Source: CAD feature listing. Evaluate the final solid. Frame: model axes, mm. Face numbers are marked on the shaded views. A direction names the side the tool comes from. Round coordinates to 2 decimals unless told otherwise and drop trailing zeros. Loops run counter-clockwise (first coordinate to the right, second up) from the corner with the lowest first, then second, coordinate; pieces in that order, holes last. Notation, with made-up numbers: M 71.5,77 L 102.5,77 A20 ccw 102.5,107 Z; hole C -4,-34 d2. An arc over 180 degrees is marked long. One line per item, written item: value.
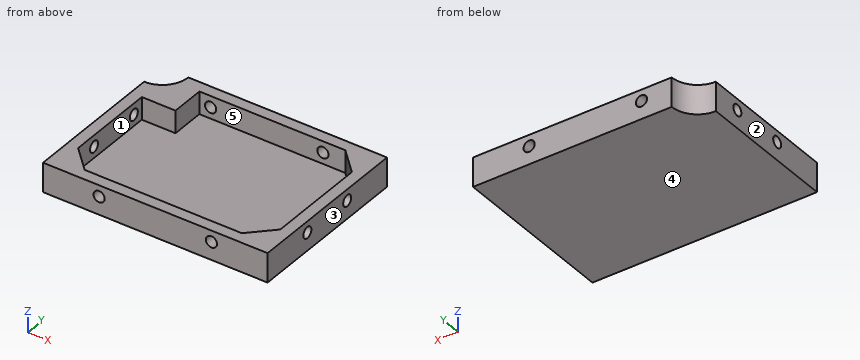
from build123d import *

# Parameters (mm, degrees)
BOSS_EXTRU_1_DEPTH        = 13
COQUE1_T                  = -5
COQUE1_THICKNESS_2_FACE_W = 90
COQUE1_THICKNESS_2_FACE_H = 65
COQUE1_THICKNESS_2_DEPTH  = 2
ENL_V_MAT_EXTRU_1_REACH   = 110.96
ESQUISSE2_R               = 2.5
ENL_V_MAT_EXTRU_2_REACH   = 95.396
ESQUISSE3_R               = 2.5
ESQUISSE4_W               = 15
ESQUISSE4_H               = 15
BOSS_EXTRU_2_DEPTH        = 10
ESQUISSE6_R               = 11.5
ENL_V_MAT_EXTRU_4_DEPTH   = 13


with BuildPart() as part:
    # Esquisse1 → Boss.-Extru.1 (new body)
    with BuildSketch(Plane.XY):
        Polygon((44.118436308, 33.728448276), (54.118436308, 33.728448276), (54.118436308, 23.728448276), (54.118436308, -41.271551724), (-45.881563692, -41.271551724), (-45.881563692, 33.728448276), align=None)
    extrude(amount=BOSS_EXTRU_1_DEPTH)

    # Coque1
    coque1_openings = [part.faces().sort_by_distance(p)[0] for p in [
        (4.118436308, -3.771551724, 13),
    ]]
    offset(amount=COQUE1_T, openings=coque1_openings, kind=Kind.INTERSECTION)

    # Coque1 thickness 2 face (on inner face of the shell) → Coque1 thickness 2 (cut)
    with BuildSketch(Plane(origin=(4.118436308, -3.771551724, 5), x_dir=(-1, 0, 0), z_dir=(0, 0, -1))):
        Rectangle(COQUE1_THICKNESS_2_FACE_W, COQUE1_THICKNESS_2_FACE_H)
    extrude(amount=COQUE1_THICKNESS_2_DEPTH, mode=Mode.SUBTRACT)

    # Enlèv. mat.-Extru.1: up to this face of the body (flat: up to its plane)
    enl_v_mat_extru_1_end = Plane(part.part.faces().sort_by_distance((54.118436308, -3.771551724, 6.5))[0])
    # Esquisse2 → Enlèv. mat.-Extru.1 (cut, up to the picked face)
    with BuildSketch(Plane.ZY.offset(45.881563692), mode=Mode.PRIVATE) as enl_v_mat_extru_1_sk1:
        with Locations(Location((8, -16.271551724, 0), (0, 0, 270))):
            Circle(ESQUISSE2_R)
    enl_v_mat_extru_1_tool1 = split(extrude(enl_v_mat_extru_1_sk1.sketch, amount=-ENL_V_MAT_EXTRU_1_REACH, mode=Mode.PRIVATE), bisect_by=enl_v_mat_extru_1_end, keep=Keep.BOTH, mode=Mode.PRIVATE)
    # Esquisse2 → Enlèv. mat.-Extru.1 (cut, up to the picked face)
    with BuildSketch(Plane.ZY.offset(45.881563692), mode=Mode.PRIVATE) as enl_v_mat_extru_1_sk2:
        with Locations(Location((8, 8.728448276, 0), (0, 0, 270))):
            Circle(ESQUISSE2_R)
    enl_v_mat_extru_1_tool2 = split(extrude(enl_v_mat_extru_1_sk2.sketch, amount=-ENL_V_MAT_EXTRU_1_REACH, mode=Mode.PRIVATE), bisect_by=enl_v_mat_extru_1_end, keep=Keep.BOTH, mode=Mode.PRIVATE)
    add(enl_v_mat_extru_1_tool1.solids().sort_by(Axis((-45.881564, -16.271552, 8), (1, 0, 0)))[0], mode=Mode.SUBTRACT)
    add(enl_v_mat_extru_1_tool2.solids().sort_by(Axis((-45.881564, 8.728448, 8), (1, 0, 0)))[0], mode=Mode.SUBTRACT)

    # Enlèv. mat.-Extru.2: up to this face of the body (flat: up to its plane)
    enl_v_mat_extru_2_end = Plane(part.part.faces().sort_by_distance((4.118436308, 33.728448276, 6.5))[0])
    # Esquisse3 → Enlèv. mat.-Extru.2 (cut, up to the picked face)
    with BuildSketch(Plane.XZ.offset(41.271551724), mode=Mode.PRIVATE) as enl_v_mat_extru_2_sk1:
        with Locations(Location((-20.881563692, 8, 0), (0, 0, 270))):
            Circle(ESQUISSE3_R)
    enl_v_mat_extru_2_tool1 = split(extrude(enl_v_mat_extru_2_sk1.sketch, amount=-ENL_V_MAT_EXTRU_2_REACH, mode=Mode.PRIVATE), bisect_by=enl_v_mat_extru_2_end, keep=Keep.BOTH, mode=Mode.PRIVATE)
    # Esquisse3 → Enlèv. mat.-Extru.2 (cut, up to the picked face)
    with BuildSketch(Plane.XZ.offset(41.271551724), mode=Mode.PRIVATE) as enl_v_mat_extru_2_sk2:
        with Locations(Location((29.118436308, 8, 0), (0, 0, 270))):
            Circle(ESQUISSE3_R)
    enl_v_mat_extru_2_tool2 = split(extrude(enl_v_mat_extru_2_sk2.sketch, amount=-ENL_V_MAT_EXTRU_2_REACH, mode=Mode.PRIVATE), bisect_by=enl_v_mat_extru_2_end, keep=Keep.BOTH, mode=Mode.PRIVATE)
    add(enl_v_mat_extru_2_tool1.solids().sort_by(Axis((-20.881564, -41.271552, 8), (0, 1, 0)))[0], mode=Mode.SUBTRACT)
    add(enl_v_mat_extru_2_tool2.solids().sort_by(Axis((29.118436, -41.271552, 8), (0, 1, 0)))[0], mode=Mode.SUBTRACT)

    # Esquisse4 → Boss.-Extru.2 (add)
    with BuildSketch(Plane.XY.offset(3)):
        Polygon((-30.881563692, -36.271551724), (-40.881563692, -26.271551724), (-40.881563692, -36.271551724), align=None)
        Polygon((49.118436308, 28.728448276), (49.118436308, 18.728448276), (39.118436308, 28.728448276), align=None)
        Polygon((49.118436308, -36.271551724), (49.118436308, -26.271551724), (39.118436308, -36.271551724), align=None)
        with Locations((-33.381563692, 21.228448276)):
            Rectangle(ESQUISSE4_W, ESQUISSE4_H)
    extrude(amount=BOSS_EXTRU_2_DEPTH)

    # Esquisse6 → Enlèv. mat.-Extru.4 (cut)
    with BuildSketch(Plane.XY.offset(13)):
        with Locations((-45.881563692, 33.728448276)):
            Circle(ESQUISSE6_R)
    extrude(amount=-ENL_V_MAT_EXTRU_4_DEPTH, mode=Mode.SUBTRACT)


solid = part.part
1. Reachability of the marked faces 4 and 5 from +Z, -Z, +X, -X, +Y, -Y: full face, straight path, thin tool, end or side. Return the list, or none.
Report:
face 4: -Z, +X, -X, +Y, -Y
face 5: +Z
2. Section query C-C (y = -7.5). Return the cut outline in (x, z), and give its area (3 significant figures).
Report:
outline: M -45.88,0 L 54.12,0 L 54.12,13 L 49.12,13 L 49.12,3 L -40.88,3 L -40.88,13 L -45.88,13 Z
area: 400 mm2
3. Section query A-A (y = 9). Return the cut outline in (x, z).
Report:
outline: M -45.88,0 L 54.12,0 L 54.12,5.51 L 49.12,5.51 L 49.12,3 L -40.88,3 L -40.88,5.51 L -45.88,5.51 Z; M -45.88,10.49 L -40.88,10.49 L -40.88,13 L -45.88,13 Z; M 49.12,10.49 L 54.12,10.49 L 54.12,13 L 49.12,13 Z
4. Ray query, line 1 (X direction, y = -40.25, z = 8); line 2 (X direction, y = -14, z = 3.25); line 3 (Y direction, x = 29.5, z = 5.25). Return the intervals inside material, ascending. Write a range as [from, to].
Report:
line 1: x = [-45.88, -23.38], [-18.38, 26.62], [31.62, 54.12]
line 2: x = [-45.88, -40.88], [49.12, 54.12]
line 3: y = [-41.27, -36.27], [28.73, 33.73]
5. Section query B-B (x = -7). Return the cut outline in (y, z).
Report:
outline: M -41.27,0 L 33.73,0 L 33.73,13 L 28.73,13 L 28.73,3 L -36.27,3 L -36.27,13 L -41.27,13 Z
6. Pin query (flat end, axial travel): pin 1 (4 mm diameter, centred on y = -16.27, z = 8, fed in from -X). Return the tip coordinate at first contact, or that it passes through.
Report:
pin 1: passes through
7. Section query D-D (z = 8). Count the separate pieces of the cut face and the enclosed holes in it, and give its area (3 significant figures).
Report:
separate pieces: 8
enclosed holes: 0
area: 1,720 mm2
8. Pull-direction query (X, two-part tool) for the marked faces 1, 2 and 3; classes: released by +X, released by -X, zero draft, split by the parting line, or undercut.
Report:
face 1: undercut
face 2: released by -X
face 3: released by +X
